Could you check a few things on this model? Use its own coordinates, in mm. Give positions to 0.01 mm unless a question says otherwise; leave off trailing zeros. Loops run counter-clockwise (first coordinate to the right, second up) from the corner with the lowest first, then second, coordinate; pieces in that order, holes last. Notation, with made-up numbers: (47.25, 11) - (69.25, 11) arc R11 ccw to (69.25, 22) - close; hole circle Ø1 at (-22, 61.25). An arc over 180 degrees is marked (long way). Write each question's results on one line, items separated by ' | '. Start each with the question number.
1) I want a section at C-C, the plane y = -3.25. Write out the boundary of the cut face in (x, z).
2) If I drill on probe 1 along X at (y, z) = (-3, 10.5); probe 2 along X at (y, z) = (3.75, 13.5); probe 3 along Y at (x, z) = (5.5, 2.75), over which ranges is the centre line in solid material (lowest first)? Write a range as [from, to].
3) I want a section at A-A, the plane z = 12. Write out the boundary of the cut face in (x, y).
4) I'm going to push flat-ended pins straight in: pin 1 (2 mm diameter, centred on x = 4, y = 2, fed in from -Z); pin 2 (1.5 mm diameter, centred on y = -2.5, z = 9.5, fed in from +X); pin 3 (2 mm diameter, centred on y = -4, z = 5.5, fed in from +X); pin 4 (1.5 mm diameter, centred on y = 2, z = 9.5, fed in from -X). Where does each tip first touch, or does it pass through?
5) I want a section at B-B, the plane x = 5. Write out the boundary of the cut face in (y, z), and give its area (3 significant figures).
6) If we mould it in two halves opening along X, with no side actions, what happens to faces 1 (the face through (-6, 0, 7)), 2 (the face through (6, 0, 7)), 3 (the face through (0, -5, 7))? For each: +X half, -X half, draft (parallel to the pull), parting line (faces both ways), or undercut.
Autodesk Inventor part; units mm, degrees
ref_plane "YZ Plane" through (0, 0, 0) normal (1, 0, 0) x (0, 1, 0)
ref_plane "XZ Plane" through (0, 0, 0) normal (0, 1, 0) x (-1, 0, 0)
ref_plane "XY Plane" through (0, 0, 0) normal (0, 0, 1) x (1, 0, 0)
sketch "Esquisse1" plane through (0, 0, 0) normal (0, 0, 1) x (1, 0, 0)
  circle A0 centre (0, 0) radius 6
  line L0 (-3.3166, 5) -> (3.3166, 5)
  line L1 (-3.3166, -5) -> (3.3166, -5)
  dimension "d0" = 12
  dimension "d1" = 10
  dimension "d2" = 5
extrude "Extrusion1" add sketch "Esquisse1" along normal blind 14 contours A0 L1 L0
fillet "Congé1" radius 0.5 4 edges at (3.3166, 5, 7) (-3.3166, 5, 7) (3.3166, -5, 7) (-3.3166, -5, 7)
properties part number "moteur" material "Acier"
Answers:
1) outline: (-5.04, 0) - (5.04, 0) - (5.04, 14) - (-5.04, 14) - close
2) probe 1: x = [-5.2, 5.2] | probe 2: x = [-4.68, 4.68] | probe 3: y = [-2.4, 2.4]
3) outline: (-3.45, -4.91) arc R0.5 ccw to (-3.16, -5) - (3.16, -5) arc R0.5 ccw to (3.45, -4.91) arc R6 ccw to (3.45, 4.91) arc R0.5 ccw to (3.16, 5) - (-3.16, 5) arc R0.5 ccw to (-3.45, 4.91) arc R6 ccw to start
4) pin 1: stops at z = 0 | pin 2: stops at x = 5.74 | pin 3: stops at x = 5.2 | pin 4: stops at x = -5.87
5) outline: (-3.32, 0) - (3.32, 0) - (3.32, 14) - (-3.32, 14) - close | area: 92.9 mm2
6) face 1: -X half | face 2: +X half | face 3: draft
